Source: CAD feature listing. Evaluate the final solid. Frame: model axes, mm. A direction names the side the tool comes from. Give positions to 0.01 mm unless a question says otherwise; leave off trailing zeros. Loops run counter-clockwise (first coordinate to the right, second up) from the corner with the lowest first, then second, coordinate; pieces in that order, holes last. Notation, with made-up numbers: (57.25, 58) - (104.25, 58) arc R19 cw to (104.25, 66) - close; hole circle Ø6 at (77.25, 59.5). An arc over 180 degrees is marked (long way). Put each result on its own line as item: value.
```python
from build123d import *

# Parameters (mm, degrees)
SKETCH1_W           = 15.875
SKETCH1_H           = 22.352
SKETCH1_R           = 2.032
SKETCH1_W_2         = 31.75
SKETCH1_H_2         = 31.75
SKETCH1_R_2         = 7.112
SKETCH1_R_3         = 1.778
BOSS_EXTRUDE1_DEPTH = 1.5875


with BuildPart() as part:
    # Sketch1 → Boss-Extrude1 (new body)
    with BuildSketch(Plane.XY):
        with Locations((-23.8125, 0)):
            Rectangle(SKETCH1_W, SKETCH1_H)
        with Locations((-25.4, 0)):
            Circle(SKETCH1_R, mode=Mode.SUBTRACT)
        Rectangle(SKETCH1_W_2, SKETCH1_H_2)
        Circle(SKETCH1_R_2, mode=Mode.SUBTRACT)
        with Locations((-10.955912468, -10.955912468)):
            Circle(SKETCH1_R_3, mode=Mode.SUBTRACT)
        with Locations((10.955912468, 10.955912468)):
            Circle(SKETCH1_R_3, mode=Mode.SUBTRACT)
        with Locations((23.8125, 0)):
            Rectangle(SKETCH1_W, SKETCH1_H)
        with Locations((25.4, 0)):
            Circle(SKETCH1_R, mode=Mode.SUBTRACT)
    extrude(amount=BOSS_EXTRUDE1_DEPTH)


solid = part.part
```
1) Mould query, pull axis X, two halves, no side actions, for faces 1 (the flat face through (-31.75, 0, 1)), 2 (the cylindrical face through (9.545, 9.874, 0.783)), 3 (the flat face through (-0.4, 7.3, 0)), 4 (the cylindrical face through (-27.01, -1.24, 0.78)). Classes: pulls with the +X half, pulls with the -X half, needs draft (parallel to the pull), parting line crosses it, or undercut.
Check result:
face 1: pulls with the -X half
face 2: undercut
face 3: needs draft
face 4: undercut
2) Pin query (flat end, axial travel): P1, Ø2.5, axis at x = 25.4, y = 0, coming from the +Z side; P2, Ø0.5, axis at y = -13.5, z = 1, coming from the -X side (3 decimals); P3, Ø0.8, axis at x = 20.5, z = 0.5, coming from the +Y side; P4, Ø0.5, axis at x = -21.5, z = 1, coming from the -Y side. Return the tip coordinate at first contact, or that it passes through.
Check result:
P1: through
P2: x = -15.875
P3: y = 11.18
P4: y = -11.18
3) Material intervals for line 1 along Y through (x, z) = (0, 1) (3 decimals); line 2 along X through (y, z) = (-0.5, 0.9); line 3 along Y through (x, z) = (17, 1.3), sorted ascending. Write a range as [from, to].
Check result:
line 1: [-15.875, -7.112], [7.112, 15.875]
line 2: [-31.75, -27.37], [-23.43, -7.09], [7.09, 23.43], [27.37, 31.75]
line 3: [-11.18, 11.18]
4) Section query B-B, the plane y = 0. Output: boundary loops of the cut face in (x, z).
Check result:
outline: (-31.75, 0) - (-27.43, 0) - (-27.43, 1.59) - (-31.75, 1.59) - close; (-23.37, 0) - (-7.11, 0) - (-7.11, 1.59) - (-23.37, 1.59) - close; (7.11, 0) - (23.37, 0) - (23.37, 1.59) - (7.11, 1.59) - close; (27.43, 0) - (31.75, 0) - (31.75, 1.59) - (27.43, 1.59) - close
5) Access query for faces 5 (the flat face through (-24, 11.176, 1)), 6 (the flat face through (31.75, 0, 1)), 7 (the flat face through (-15.875, -14, 1)), 8 (the flat face through (24, 11.176, 1)), 9 (the flat face through (15.875, -14, 1)). Directions: +Z, -Z, +X, -X, +Y, -Y. A direction counts if a zero-diameter tool reaches every point of the face in a straight line with its end or side. Return the directions, or none.
Check result:
face 5: +Z, -Z, -X, +Y
face 6: +Z, -Z, +X, +Y, -Y
face 7: +Z, -Z, -X, -Y
face 8: +Z, -Z, +X, +Y
face 9: +Z, -Z, +X, -Y
6) Section query D-D, the plane x = 0. Output: boundary loops of the cut face in (y, z) (1 decimal).
Check result:
outline: (-15.9, 0) - (-7.1, 0) - (-7.1, 1.6) - (-15.9, 1.6) - close; (7.1, 0) - (15.9, 0) - (15.9, 1.6) - (7.1, 1.6) - close
7) Section query A-A, the plane x = -25.4. Output: boundary loops of the cut face in (y, z).
Check result:
outline: (-11.18, 0) - (-2.03, 0) - (-2.03, 1.59) - (-11.18, 1.59) - close; (2.03, 0) - (11.18, 0) - (11.18, 1.59) - (2.03, 1.59) - close
8) Section query C-C, the plane z = 0.95. Output: boundary loops of the cut face in (x, y) (3 decimals), plus the area to 3 significant figures.
Check result:
outline: (-31.75, -11.176) - (-15.875, -11.176) - (-15.875, -15.875) - (15.875, -15.875) - (15.875, -11.176) - (31.75, -11.176) - (31.75, 11.176) - (15.875, 11.176) - (15.875, 15.875) - (-15.875, 15.875) - (-15.875, 11.176) - (-31.75, 11.176) - close; hole circle Ø4.064 at (-25.4, 0); hole circle Ø3.556 at (-10.956, -10.956); hole circle Ø14.224 at (0, 0); hole circle Ø3.556 at (10.956, 10.956); hole circle Ø4.064 at (25.4, 0)
area: 1,510 mm²
